Input: part model. Units: mm. Frame: model coordinates. A direction names the side the tool comes from. Give positions to 0.01 mm unless a question says otherwise; leave off trailing zeros. Loops run counter-clockwise (first coordinate to the right, second up) from the corner with the lowest first, then second, coordinate; pieces in that order, holes last. Notation, with made-up numbers: (28.5, -22.75) - (84.5, -22.75) arc R20 cw to (84.5, 2.25) - close; hole circle Ø5 at (51.25, 2). An arc over 180 degrees is marked (long way). One line per question, with ' | ' between items. Start each with the question number.
Autodesk Inventor part; units mm, degrees
ref_plane "YZ Plane" through (0, 0, 0) normal (1, 0, 0) x (0, 1, 0)
ref_plane "XZ Plane" through (0, 0, 0) normal (0, 1, 0) x (-1, 0, 0)
ref_plane "XY Plane" through (0, 0, 0) normal (0, 0, 1) x (1, 0, 0)
sketch "Sketch1" plane through (0, 0, 0) normal (0, 0, 1) x (1, 0, 0)
  line L0 (-15.405, 0) -> (15.405, 0)
  line L1 (15.405, 0) -> (15.405, 3.6)
  line L2 (15.405, 3.6) -> (8.48, 3.6)
  line L3 (8.48, 3.6) -> (8.48, 9.96)
  line L4 (8.48, 9.96) -> (-8.48, 9.96)
  line L5 (-8.48, 9.96) -> (-8.48, 3.6)
  line L6 (-8.48, 3.6) -> (-15.405, 3.6)
  line L7 (-15.405, 3.6) -> (-15.405, 0)
  point P0 (0, 0)
  point P1 (0, 0)
  dimension "d0" = 16.96
  dimension "d1" = 9.96
  dimension "d2" = 3.6
  dimension "d3" = 30.81
extrude "Extrusion1" add sketch "Sketch1" along normal blind 0.0001
sketch "Sketch2" plane through (0, 0, 0) normal (0, 0, -1) x (-1, 0, 0)
  line L0 (15.405, 3.6) -> (15.405, 0)
  line L1 (-15.405, 0) -> (15.405, 0)
  line L2 (15.405, 0) -> (15.405, 12.58)
  line L3 (15.405, 12.58) -> (-15.405, 12.58)
  line L4 (-15.405, 12.58) -> (-15.405, 0)
  dimension "d6" = 12.58
extrude "Extrusion2" add sketch "Sketch2" along normal blind 3.6
sketch "Sketch5" plane through (0, 0, -3.6) normal (0, 0, -1) x (-1, 0, 0)
  line L0 (15.405, 0) -> (-15.405, 0)
  line L1 (-15.405, 12.58) -> (15.405, 12.58)
  line L2 (-7.4102, 10.415) -> (7.4102, 10.415)
  line L3 (8.395, 9.2414) -> (7.293, 2.9914)
  line L4 (6.3081, 2.165) -> (-6.3081, 2.165)
  line L5 (-7.293, 2.9914) -> (-8.395, 9.2414)
  arc A0 (-7.4102, 10.415) -> (-8.395, 9.2414) centre (-7.4102, 9.415) ccw
  arc A1 (8.395, 9.2414) -> (7.4102, 10.415) centre (7.4102, 9.415) ccw
  arc A2 (-7.293, 2.9914) -> (-6.3081, 2.165) centre (-6.3081, 3.165) ccw
  arc A3 (6.3081, 2.165) -> (7.293, 2.9914) centre (6.3081, 3.165) ccw
  line L6 (0, 12.58) -> (0, 0) construction
  line L7 (0, 10.415) -> (0, 12.58) construction
  line L8 (0, 0) -> (0, 2.165) construction
  arc A4 (-7.4102, 10.915) -> (-8.8874, 9.1545) centre (-7.4102, 9.415) ccw
  line L9 (-7.4102, 10.915) -> (7.4102, 10.915)
  arc A5 (8.8874, 9.1545) -> (7.4102, 10.915) centre (7.4102, 9.415) ccw
  line L10 (8.8874, 9.1545) -> (7.7854, 2.9045)
  arc A6 (6.3081, 1.665) -> (7.7854, 2.9045) centre (6.3081, 3.165) ccw
  line L11 (6.3081, 1.665) -> (-6.3081, 1.665)
  arc A7 (-7.7854, 2.9045) -> (-6.3081, 1.665) centre (-6.3081, 3.165) ccw
  line L12 (-7.7854, 2.9045) -> (-8.8874, 9.1545)
  dimension "d22" = 100
  dimension "d23" = 100
  dimension "d24" = 1
  dimension "d25" = 1
  dimension "d26" = 8.25
  dimension "d27" = 16.79
  dimension "d29" = 0.5
extrude "Extrusion3" add sketch "Sketch5" along normal blind 5.9
sketch "Sketch6" plane through (0, 0, -3.6) normal (0, 0, -1) x (-1, 0, 0)
  line L0 (-15.405, 0) -> (-15.405, 12.58)
  line L1 (15.405, 0) -> (-15.405, 0)
  line L2 (15.405, 12.58) -> (15.405, 0)
  line L3 (-15.405, 12.58) -> (15.405, 12.58)
  line L4 (-7.4102, 10.915) -> (7.4102, 10.915)
  arc A0 (8.8874, 9.1545) -> (7.4102, 10.915) centre (7.4102, 9.415) ccw
  line L5 (8.8874, 9.1545) -> (7.7854, 2.9045)
  arc A1 (6.3081, 1.665) -> (7.7854, 2.9045) centre (6.3081, 3.165) ccw
  line L6 (6.3081, 1.665) -> (-6.3081, 1.665)
  arc A2 (-7.7854, 2.9045) -> (-6.3081, 1.665) centre (-6.3081, 3.165) ccw
  line L7 (-7.7854, 2.9045) -> (-8.8874, 9.1545)
  arc A3 (-7.4102, 10.915) -> (-8.8874, 9.1545) centre (-7.4102, 9.415) ccw
  line L8 (-15.155, 11.83) -> (-15.155, 0.75)
  line L9 (-14.655, 0.25) -> (14.655, 0.25)
  line L10 (15.155, 0.75) -> (15.155, 11.83)
  line L11 (14.655, 12.33) -> (-14.655, 12.33)
  line L12 (-8.395, 9.2414) -> (-7.293, 2.9914)
  arc A4 (-7.293, 2.9914) -> (-6.3081, 2.165) centre (-6.3081, 3.165) ccw
  line L13 (-6.3081, 2.165) -> (6.3081, 2.165)
  arc A5 (-14.655, 12.33) -> (-15.155, 11.83) centre (-14.655, 11.83) ccw
  arc A6 (15.155, 11.83) -> (14.655, 12.33) centre (14.655, 11.83) ccw
  arc A7 (14.655, 0.25) -> (15.155, 0.75) centre (14.655, 0.75) ccw
  arc A8 (-15.155, 0.75) -> (-14.655, 0.25) centre (-14.655, 0.75) ccw
  dimension "d32" = 0.25
  dimension "d33" = 0.5
extrude "Extrusion4" add sketch "Sketch6" along normal blind 0.5 contours A5 L11 A6 L10 A7 L9 A8 L8
sketch "Sketch7" plane through (0, 0, -4.1) normal (0, 0, -1) x (-1, 0, 0)
  line L0 (-14.655, 12.33) -> (14.655, 12.33)
  line L1 (14.655, 0.25) -> (-14.655, 0.25)
  circle A0 centre (12.495, 6.29) radius 2.25
  line L2 (12.495, 6.29) -> (12.495, 12.33)
  line L3 (12.495, 6.29) -> (12.495, 0.25)
  line L4 (15.405, 12.58) -> (15.405, 0)
  dimension "d36" = 4.5
  dimension "d37" = 2.91
extrude "Extrusion5" add sketch "Sketch7" along normal blind 5.4
sketch "Sketch8" plane through (-12.495, 6.29, -9.5) normal (0, 0, -1) x (-1, 0, 0)
  circle A0 centre (0, 0) radius 2.25
hole "Hole2" at (-12.495, 6.29, -9.5) direction (0, 0, 1) diameter 2.156 end through all
chamfer "Chamfer2" distance 0.25 angle 45 2 edges at (-10.245, 6.29, -9.5) (-12.495, 5.212, -9.5)
mirror "Mirror2" about plane through (0, 0, 0) normal (1, 0, 0) of "Extrusion5", "Hole2", "Chamfer2"
sketch "Sketch9" plane through (0, 0, -3.6) normal (0, 0, -1) x (-1, 0, 0)
  line L0 (7.4102, 10.415) -> (-7.4102, 10.415)
  line L1 (-6.3081, 2.165) -> (6.3081, 2.165)
  line L2 (0, 2.165) -> (0, 10.415) construction
  line L3 (-1.7032, 7.71) -> (6.4948, 7.71) construction
  line L4 (-1.5161, 4.87) -> (6.4574, 4.87) construction
  line L5 (-1.7032, 7.71) -> (-1.7032, 10.415) construction
  line L6 (-1.5161, 4.87) -> (-1.5161, 2.165) construction
  line L7 (-1.37, 8.1856) -> (-1.37, 4.0304) construction
  circle A0 centre (0, 7.71) radius 0.335
  circle A1 centre (-1.37, 4.87) radius 0.335
  circle A2 centre (2.74, 7.71) radius 0.335
  circle A3 centre (1.37, 4.87) radius 0.335
  circle A4 centre (5.48, 7.71) radius 0.335
  circle A5 centre (4.11, 4.87) radius 0.335
  dimension "d49" = 2.84
  dimension "d50" = 1.37
  dimension "d51" = 0.67
  dimension "d54" = 2.74
extrude "Extrusion6" add sketch "Sketch9" along normal blind 5
mirror "Mirror3" about plane through (0, 0, 0) normal (1, 0, 0) of "Extrusion6"
properties part number "cRIO-FRC 9M D-Shell" material "ABS Plastic"
Q1. Draft query along Y for faces 4 (the face through (-10.247, 6.191, -6.639)), 5 (the face through (0, 0, -2)), 6 (the face through (0, 6, -3.6)). Return one class per face: +Y half, -Y half, draft (parallel to the pull), parting line (faces both ways), or undercut.
Q2. Section A-A, the plane z = -4.75. Count the separate pieces of the cut face and the enclosed holes in it, plus the area to 3 significant figures.
Q3. Line query: L1, parallel to X at y = 6.29, z = -2 (3 decimals); L2, parallel to Y at x = 5.5, z = -6 (3 decimals); L3, parallel to X at y = 6.29, z = -4.5 (3 decimals). Output: solid intervals per line, ascending. Write a range as from..to.
Q4. Access query for faces 1 (the face through (-8.344, 6.073, -6.762)), 2 (the face through (10.71, 4.92, -6.64)), 3 (the face through (12.448, 5.213, -4.56)). Directions: +Z, -Z, +X, -X, +Y, -Y. A direction counts if a zero-diameter tool reaches every point of the face in a straight line with its end or side. Return the directions, or none.
Q5. Section C-C, the plane z = -3. Output: boundary loops of the cut face in (x, y) (3 decimals), plus the area to 3 significant figures.
Q6. First-contact query: pin 1 (0.7 mm diameter, centred on x = -5.5, y = 7.5, fed in from -Z); pin 2 (3 mm diameter, centred on x = -1.5, z = -8, fed in from +Y) (3 decimals); pin 3 (1 mm diameter, centred on y = 6.5, z = -7.5, fed in from +X) (3 decimals). Flat tips, straight axial feed; report the tip coordinate or a pass-through.
Solved:
1) face 4: parting line | face 5: -Y half | face 6: undercut
2) separate pieces: 12 | enclosed holes: 3 | area: 51.7 mm²
3) L1: x = -15.405..-13.573, -11.417..11.417, 13.573..15.405 | L2: y = 1.665..2.165, 7.376..8.044, 10.415..10.915 | L3: x = -14.745..-13.573, -11.417..-10.245, -8.382..-7.875, 7.875..8.382, 10.245..11.417, 13.573..14.745
4) face 1: -Z, -Y | face 2: -Z | face 3: +Z, -Z
5) outline: (-15.405, 0) - (15.405, 0) - (15.405, 12.58) - (-15.405, 12.58) - close; hole circle Ø2.156 at (-12.495, 6.29); hole circle Ø2.156 at (12.495, 6.29) | area: 380 mm²
6) pin 1: stops at z = -8.6 | pin 2: stops at y = 10.915 | pin 3: stops at x = 14.745
